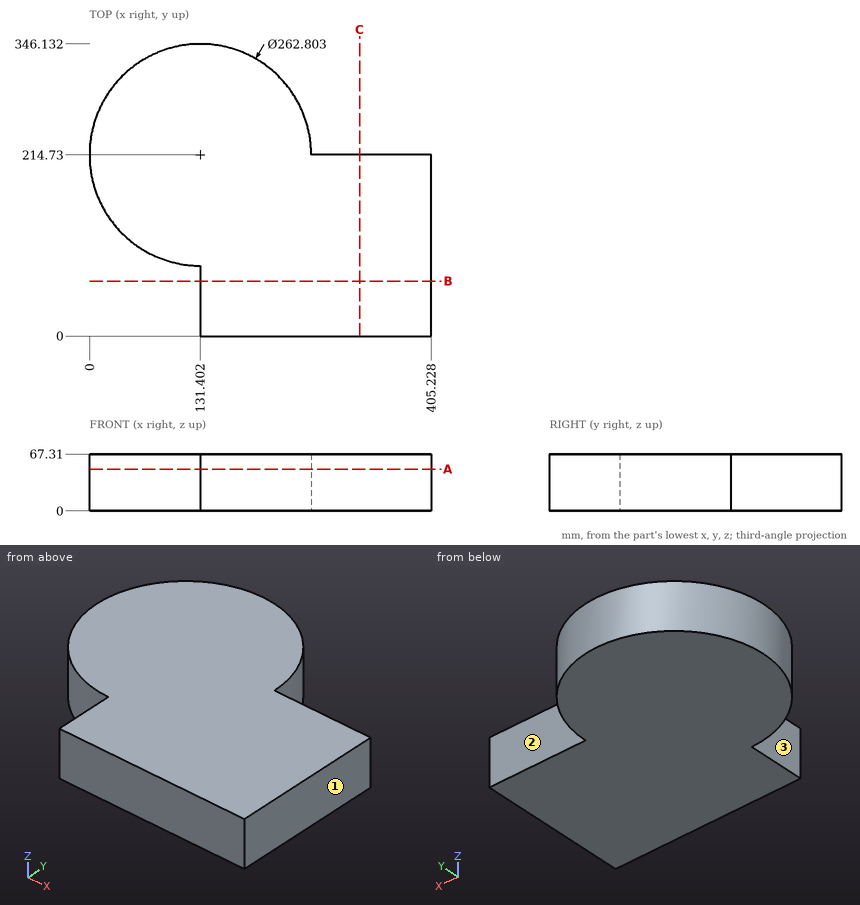
Here's the drawing with two shaded views (mm, measured from the low corner). I have some questions. A direction names the side the tool comes from. Give positions to 0.01 mm unless a question says otherwise; leave off trailing zeros. Order: outer loops, then holes, each group sorted by start corner. A loop starts at its lowest first (then second) coordinate and runs counter-clockwise, first axis right, second up.
Q1. For the marked faces 1, 2 and 3, which set-ups out of +Z, -Z, +X, -X, +Y, -Y let a thin tool reach every point of the face, with its end or its side?
Q2. Suppose I cut it at B-B, the plane y = 65. Write out the boundary of the cut face in (x, z).
Q3. Suppose I cut it at A-A, the plane z = 49.5. Write out the boundary of the cut face in (x, y), and give its area (3 significant figures).
Q4. If I drill on line 1 along X through (y, z) = (73.5, 13); line 2 along Y through (x, z) = (127.5, 23); line 3 along X through (y, z) = (219, 11), over which ranges is the centre line in solid material (lowest first)?
Q5. Suppose I cut it at C-C, the plane x = 320. Write out the boundary of the cut face in (y, z), and give its area (3 significant figures).
Q6. I'm going to push flat-ended pins straight in: P1, Ø3, axis at y = 232, z = 24, coming from the -X side; P2, Ø8, axis at y = 125, z = 25.5, coming from the -X side; P3, Ø5, axis at y = 105, z = 57.5, coming from the -X side (1 decimal). Where does each tip first touch, or does it pass through?
Solution:
1. face 1: +Z, -Z, +X, +Y, -Y
1. face 2: +Z, -Z, +X, +Y
1. face 3: +Z, -Z, -X, -Y
2. outline: (131.4, 0) - (405.23, 0) - (405.23, 67.31) - (131.4, 67.31) - close
3. outline: (131.4, 0) - (405.23, 0) - (405.23, 214.73) - (262.8, 214.73) arc R131.4 ccw (long way) to (131.4, 83.33) - close
3. area: 99,500 mm2
4. line 1: x = 131.4 to 405.23
4. line 2: y = 83.39 to 346.07
4. line 3: x = 0.07 to 262.73
5. outline: (0, 0) - (214.73, 0) - (214.73, 67.31) - (0, 67.31) - close
5. area: 14,500 mm2
6. P1: stops at x = 0.95
6. P2: stops at x = 31.82
6. P3: stops at x = 55.5
